Work out the finished part from the listing and answer in its coordinate system (mm). A direction names the side the tool comes from. Give positions to 0.01 mm unless a question says otherwise; leave off trailing zeros. Loops run counter-clockwise (first coordinate to the right, second up) from the corner with the lowest first, then second, coordinate; pieces in that order, holes last. Notation, with made-up numbers: M 63.5,-39 L 92.5,-39 A32 ccw 92.5,-4 Z; hole C 30,-4 d6. An arc over 180 degrees is marked long. Answer as a JSON object with one key per item and string values. Group by question number.
```python
from build123d import *

# Parameters (mm, degrees)
BOSS_EXTRUDE1_DEPTH     = 46.1
CUT_EXTRUDE1_START      = -8
CUT_EXTRUDE1_DEPTH      = 35.707069821
SKETCH3_R               = 5
CUT_EXTRUDE2_DEPTH      = 4.2
SKETCH4_R               = 3
CUT_EXTRUDE3_DEPTH      = 118.073974259
CUT_EXTRUDE4_START      = -33.042265264
CUT_EXTRUDE4_DEPTH      = 39.042265264
CUT_EXTRUDE4_START_2    = 14
CUT_EXTRUDE4_2_DEPTH    = 32.1
CUT_EXTRUDE4_START_3    = -47.726546034
CUT_EXTRUDE4_3_DEPTH    = 7.708156307
SKETCH8_W               = 31
SKETCH8_H               = 27.1
CUT_EXTRUDE5_DEPTH      = 119.273474775
SKETCH9_W               = 8
SKETCH9_H               = 25
BOSS_EXTRUDE2_DEPTH     = 19
SKETCH10_R              = 7.1
CUT_EXTRUDE6_DEPTH      = 119.273474775
SKETCH11_R              = 7.6
CUT_EXTRUDE7_DEPTH      = 1.2
CUT_EXTRUDE8_DEPTH      = 119.273474775
CUT_EXTRUDE8_DEPTH_BACK = 119.273474775
SKETCH12_R              = 2.1
CUT_EXTRUDE9_DEPTH      = 4.2
CUT_EXTRUDE9_DEPTH_BACK = 119.273474775
CUT_EXTRUDE9_START      = -8
SKETCH14_R              = 4
SKETCH14_R_2            = 2.1
CUT_EXTRUDE10_START     = -24
SKETCH14_3_R            = 4
CUT_EXTRUDE10_DEPTH     = 4.2
FILLET13_R              = 10
FILLET14_R              = 1


with BuildPart() as part:
    # Sketch1 → Boss-Extrude1 (new body)
    with BuildSketch(Plane(origin=(0, 0, 0), x_dir=(1, 0, 0), z_dir=(0, 1, 0))):
        with BuildLine():
            Line((0, 0), (8, 0))
            Line((8, 0), (8, -52.240297657))
            ThreePointArc((8, -52.240297657), (7.396926208, -55.660499091), (5.660444431, -58.668173754))
            Line((5.660444431, -58.668173754), (-19.707069821, -88.9))
            Line((-19.707069821, -88.9), (-19.707069821, -102.9))
            Line((-19.707069821, -102.9), (-27.707069821, -102.9))
            Line((-27.707069821, -102.9), (-27.707069821, -88.9))
            Line((-27.707069821, -88.9), (-2.339555569, -58.668173754))
            ThreePointArc((-2.339555569, -58.668173754), (-0.603073792, -55.660499091), (0, -52.240297657))
            Line((0, -52.240297657), (0, 0))
        make_face()
    extrude(amount=BOSS_EXTRUDE1_DEPTH)

    # Cut-Extrude1: read off the stored shape, not the designer's step
    # Cut-Extrude1 outline → Cut-Extrude1 (cut)
    with BuildSketch(Plane(origin=(-19.707069821, 0, 0), x_dir=(0, 0, -1), z_dir=(1, 0, 0)).offset(CUT_EXTRUDE1_START)):
        with BuildLine():
            ThreePointArc((-95.9, 0), (-100.849747468, 2.050252532), (-102.9, 7))
            Line((-102.9, 7), (-102.9, 0))
            Line((-102.9, 0), (-95.9, 0))
        make_face()
        with BuildLine():
            ThreePointArc((-102.9, 7), (-100.849747468, 11.949747468), (-95.9, 14))
            Line((-95.9, 14), (-88.9, 14))
            Line((-88.9, 14), (-88.852375001, 46.1))
            Line((-88.852375001, 46.1), (-102.9, 46.1))
            Line((-102.9, 46.1), (-102.9, 7))
        make_face()
    extrude(amount=CUT_EXTRUDE1_DEPTH, mode=Mode.SUBTRACT)

    # Sketch3 → Cut-Extrude2 (cut)
    with BuildSketch(Plane.ZY.offset(27.707069821)):
        with Locations((95.9, 7)):
            Circle(SKETCH3_R)
    extrude(amount=-CUT_EXTRUDE2_DEPTH, mode=Mode.SUBTRACT)

    # Sketch4 → Cut-Extrude3 (cut, through all)
    with BuildSketch(Plane.ZY.offset(23.507069821)):
        with Locations((95.9, 7)):
            Circle(SKETCH4_R)
    extrude(amount=-CUT_EXTRUDE3_DEPTH, mode=Mode.SUBTRACT)

    # Cut-Extrude4: read off the stored shape, not the designer's step
    # Cut-Extrude4 outline → Cut-Extrude4 (cut)
    with BuildSketch(Plane(origin=(-51.917191151, 0, 61.872499072), x_dir=(0.7660444431189772, 0, 0.6427876096865404), z_dir=(-0.6427876096865403, 0, 0.7660444431189771)).offset(CUT_EXTRUDE4_START)):
        Polygon((35.918971629, 46.1), (35.918971629, 14), (40.047327174, 46.1), align=None)
    extrude(amount=CUT_EXTRUDE4_DEPTH, mode=Mode.SUBTRACT)

    # Cut-Extrude4 2 outline → Cut-Extrude4 2 (cut)
    with BuildSketch(Plane(origin=(0, 0, 0), x_dir=(1, 0, 0), z_dir=(0, 1, 0)).offset(CUT_EXTRUDE4_START_2)):
        with BuildLine():
            Line((-3.162503825, -59.648925294), (0, -62.302581087))
            Line((0, -62.302581087), (0, -52.240297657))
            ThreePointArc((0, -52.240297657), (-0.603073792, -55.66049909), (-2.339555569, -58.668173754))
            Line((-2.339555569, -58.668173754), (-3.162503825, -59.648925294))
        make_face()
    extrude(amount=CUT_EXTRUDE4_2_DEPTH, mode=Mode.SUBTRACT)

    # Cut-Extrude4 3 outline → Cut-Extrude4 3 (add)
    with BuildSketch(Plane(origin=(0, 0, 0), x_dir=(0.7660444431189768, 0, 0.6427876096865408), z_dir=(0.6427876096865408, 0, -0.7660444431189768)).offset(CUT_EXTRUDE4_START_3)):
        Polygon((40.047327174, -46.1), (40.047327174, -14), (35.918971629, -14), align=None)
    extrude(amount=CUT_EXTRUDE4_3_DEPTH)

    # Sketch8 → Cut-Extrude5 (cut, through all)
    with BuildSketch(Plane(origin=(8, 0, 0), x_dir=(0, 0, -1), z_dir=(1, 0, 0))):
        with Locations((-15.5, 32.55)):
            Rectangle(SKETCH8_W, SKETCH8_H)
    extrude(amount=-CUT_EXTRUDE5_DEPTH, mode=Mode.SUBTRACT)

    # Sketch9 → Boss-Extrude2 (add)
    with BuildSketch(Plane(origin=(0, 0, 0), x_dir=(1, 0, 0), z_dir=(0, 1, 0))):
        with Locations((4, 12.5)):
            Rectangle(SKETCH9_W, SKETCH9_H)
    extrude(amount=BOSS_EXTRUDE2_DEPTH)

    # Sketch10 → Cut-Extrude6 (cut, through all)
    with BuildSketch(Plane(origin=(8, 0, 0), x_dir=(0, 0, -1), z_dir=(1, 0, 0))):
        with BuildLine():
            ThreePointArc((25, 3.947892292), (23.353975422, 1.740233099), (21.219790616, 0))
            Line((21.219790616, 0), (25, 0))
            Line((25, 0), (25, 3.947892292))
        make_face()
        with BuildLine():
            ThreePointArc((21.286823186, 18.957545444), (23.381362589, 17.231063475), (25, 15.052107708))
            Line((25, 15.052107708), (25, 19))
            Line((25, 19), (21.313922252, 19))
            Line((21.313922252, 19), (21.286823186, 18.957545444))
        make_face()
        with Locations((15.25, 9.5)):
            Circle(SKETCH10_R)
    extrude(amount=-CUT_EXTRUDE6_DEPTH, mode=Mode.SUBTRACT)

    # Sketch11 → Cut-Extrude7 (cut)
    with BuildSketch(Plane(origin=(8, 0, 0), x_dir=(0, 0, -1), z_dir=(1, 0, 0))):
        with Locations((15.25, 9.5)):
            Circle(SKETCH11_R)
    extrude(amount=-CUT_EXTRUDE7_DEPTH, mode=Mode.SUBTRACT)

    # Sketch12 → Cut-Extrude8 (cut, two sides: drawn at the far end of the back side and taken through both)
    with BuildSketch(Plane(origin=(8, 0, 0), x_dir=(0, 0, -1), z_dir=(1, 0, 0)).offset(-CUT_EXTRUDE8_DEPTH_BACK)):
        with Locations((-70.9, 5)):
            Circle(SKETCH12_R)
        with Locations((-10.9, 5)):
            Circle(SKETCH12_R)
    extrude(amount=CUT_EXTRUDE8_DEPTH + CUT_EXTRUDE8_DEPTH_BACK, mode=Mode.SUBTRACT)

    # Sketch14 → Cut-Extrude9 (cut, two sides: drawn at the far end of the back side and taken through both)
    with BuildSketch(Plane(origin=(8, 0, 0), x_dir=(0, 0, -1), z_dir=(1, 0, 0)).offset(CUT_EXTRUDE9_START - CUT_EXTRUDE9_DEPTH_BACK)):
        with Locations((-10.9, 5)):
            Circle(SKETCH14_R)
        with Locations((-10.9, 5)):
            Circle(SKETCH14_R_2, mode=Mode.SUBTRACT)
    extrude(amount=CUT_EXTRUDE9_DEPTH + CUT_EXTRUDE9_DEPTH_BACK, mode=Mode.SUBTRACT)

    # Sketch14<3> → Cut-Extrude10 (cut)
    with BuildSketch(Plane(origin=(8, 0, 0), x_dir=(0, 0, -1), z_dir=(1, 0, 0)).offset(CUT_EXTRUDE10_START)):
        with Locations((-70.9, 5)):
            Circle(SKETCH14_3_R)
    extrude(amount=CUT_EXTRUDE10_DEPTH, mode=Mode.SUBTRACT)

    # Fillet13
    # the kernel refuses this fillet: 10 mm, written as the material it adds along each edge
    with BuildSketch(Plane(origin=(-27.707069821, 14, 88.9), x_dir=(0, 0.9999988994008282, -0.0014836431957626689), z_dir=(1, 0, 0))) as fillet13_piece_1_section:
        with BuildLine():
            CenterArc((9.720956062, 10), FILLET13_R, 190.199837756, 79.800162244)
            Line((-0.121005032, 8.229180466), (-1.105201142, 8.052098513))
            ThreePointArc((-1.105201142, 8.052098513), (-1.010384402, 6.998508652), (-0.999998899, -0.001483643))
            Line((-0.999998899, -0.001483643), (0, -1))
            Line((0, -1), (9.720956062, -1))
            Line((9.720956062, -1), (9.720956062, 0))
        make_face()
    fillet13_piece_1 = extrude(amount=8, mode=Mode.PRIVATE)
    fillet13_piece_1 = split(fillet13_piece_1, bisect_by=Plane(origin=(-27.707069822, 14, 88.9), z_dir=(0.75978665319281, -0.12755860295201663, 0.6375367004675092)), keep=Keep.TOP, mode=Mode.PRIVATE)
    fillet13_piece_1 = split(fillet13_piece_1, bisect_by=Plane(origin=(-27.707069821, 14, 88.9), z_dir=(0.7660444431189771, 0, 0.6427876096865404)), keep=Keep.TOP, mode=Mode.PRIVATE)
    fillet13_piece_1 = split(fillet13_piece_1, bisect_by=Plane(origin=(-23.012477111, 14, 92.839231012), z_dir=(-0.7660444431189769, 0, -0.6427876096865407)), keep=Keep.TOP, mode=Mode.PRIVATE)
    add(fillet13_piece_1)
    with BuildSketch(Plane(origin=(-27.707069821, 14, 88.9), x_dir=(0, 0.9999988994008282, -0.0014836431957626689), z_dir=(1, 0, 0))) as fillet13_piece_2_section:
        with BuildLine():
            CenterArc((9.720956062, 10), FILLET13_R, 190.199837756, 79.800162244)
            Line((-0.121005032, 8.229180466), (-1.105201142, 8.052098513))
            ThreePointArc((-1.105201142, 8.052098513), (-1.010384402, 6.998508652), (-0.999998899, -0.001483643))
            Line((-0.999998899, -0.001483643), (0, -1))
            Line((0, -1), (9.720956062, -1))
            Line((9.720956062, -1), (9.720956062, 0))
        make_face()
    fillet13_piece_2 = extrude(amount=8, mode=Mode.PRIVATE)
    fillet13_piece_2 = split(fillet13_piece_2, bisect_by=Plane(origin=(-23.012477111, 14, 92.839231012), z_dir=(0.7660444431189769, 0, 0.6427876096865407)), keep=Keep.TOP, mode=Mode.PRIVATE)
    add(fillet13_piece_2)
    with BuildSketch(Plane(origin=(-27.707069821, 14, 88.9), x_dir=(0, 0.9999988994008282, -0.0014836431957626689), z_dir=(1, 0, 0))) as fillet13_piece_3_section:
        with BuildLine():
            CenterArc((9.720956062, 10), FILLET13_R, 190.199837756, 79.800162244)
            Line((-0.121005032, 8.229180466), (-1.105201142, 8.052098513))
            ThreePointArc((-1.105201142, 8.052098513), (-1.010384402, 6.998508652), (-0.999998899, -0.001483643))
            Line((-0.999998899, -0.001483643), (0, -1))
            Line((0, -1), (9.720956062, -1))
            Line((9.720956062, -1), (9.720956062, 0))
        make_face()
    fillet13_piece_3 = extrude(amount=32.302390155, mode=Mode.PRIVATE)
    fillet13_piece_3 = split(fillet13_piece_3, bisect_by=Plane(origin=(-19.707069821, 14, 88.9), z_dir=(1, 0, 0)), keep=Keep.TOP, mode=Mode.PRIVATE)
    fillet13_piece_3 = split(fillet13_piece_3, bisect_by=Plane(origin=(-23.012477111, 14, 92.839231012), z_dir=(-0.7660444431189769, 0, -0.6427876096865407)), keep=Keep.TOP, mode=Mode.PRIVATE)
    add(fillet13_piece_3)

    # Fillet14
    # the kernel refuses this fillet: 1 mm, written as the material it takes off along each edge
    with BuildSketch(Plane(origin=(6.8, 9.5, -15.25), x_dir=(0, 0, -1), z_dir=(0, -1, 0))) as fillet14_piece_1:
        with BuildLine():
            CenterArc((8.1, -0.866025404), FILLET14_R, 120, 60)
            Line((7.1, -0.866025404), (7.08, -0.866025404))
            Line((7.08, -0.866025404), (7.08, 0))
            Line((7.08, 0), (7.1, 0.02))
            ThreePointArc((7.1, 0.02), (7.35, 0.02), (7.59, 0.017320508))
            Line((7.59, 0.017320508), (7.6, 0))
        make_face()
    revolve(axis=Axis((6.8, 9.5, -15.25), (1, 0, 0)), mode=Mode.SUBTRACT)


solid = part.part
```
Item 1: A cutting plane is placed at A-A (z = 10.9). Determine the outline of the cut face in (x, y).
Item 2: For a pull along Z with two mould halves and no side action, classify faces 5 (the cylindrical face through (3.01, 2.57, -13.71)), 6 (the flat face through (2, 0, 37)), 7 (the cylindrical face through (7.414, 22.727, 55.615)) as pulls with the +Z half, pulls with the -Z half, needs draft (parallel to the pull), parting line crosses it, or undercut.
Item 3: A cutting plane is placed at D-D (x = -17.5). Determine the outline of the cut face in (y, z).
Item 4: Find the intervals of material crossed by probe 1 along Y at (x, z) = (1.5, -15.25); probe 2 along Z at (x, y) = (6.05, 5); probe 3 along Z at (x, y) = (1.45, 5), in increasing order. Write a range as [from, to].
Item 5: A tool of negligible diameter and unlimited length cuts with its end or side. For faces 1 (the flat face through (-0.4, 14, 55.7)), 2 (the flat face through (4, 32, 31)), 3 (the flat face through (-19.707, 9, 93)), 4 (the cylindrical face through (2.071, 1.095, 11.767)), from which of +Z, -Z, +X, -X, +Y, -Y can it reach the whole face along a straight path? Write none if from no direction.
Item 6: A cutting plane is placed at C-C (z = -15.25). Determine the outline of the cut face in (x, y).
Item 7: Given pin 1 Ø3 at (x, y) = (1.5, 23) entering from +Z; pin 2 Ø9 at (y, z) = (7, 95.9) entering from -X; pin 3 Ø2.5 at (y, z) = (6, 10) entering from -X, each flat-ended and moving along its own axis, determine where each tip first touches the part or whether it passes through.
Item 8: A cutting plane is placed at B-B (y = 31). Determine the outline of the cut face in (x, z).
The answers:
{
 "1": {"outline": "M 0,0 L 8,0 L 8,2.9 L 4.2,2.9 L 4.2,1 L 0,1 Z; M 0,9 L 4.2,9 L 4.2,7.1 L 8,7.1 L 8,19 L 0,19 Z"},
 "2": {"face 5": "undercut", "face 6": "needs draft", "face 7": "pulls with the +Z half"},
 "3": {"outline": "M 0,76.74 L 14,76.74 L 46.1,83.16 L 46.1,86.27 L 0,86.27 Z"},
 "4": {"probe 1": "y = [0, 2.4], [16.6, 19]", "probe 2": "z = [-25, -20.75], [-9.75, 8.8], [13, 58.17]", "probe 3": "z = [-25, -20.74], [-9.76, 6.9], [14.9, 63.69]"},
 "5": {"face 1": "-Z, -X, +Y", "face 2": "-Z, +X, -X, +Y", "face 3": "+Z, +X, +Y, -Y", "face 4": "-X"},
 "6": {"outline": "M 0,0 L 8,0 L 8,1.9 L 6.8,1.9 A1 ccw 5.93,2.4 L 0,2.4 Z; M 0,16.6 L 5.93,16.6 A1 ccw 6.8,17.1 L 8,17.1 L 8,19 L 0,19 Z"},
 "7": {"pin 1": "stops at z = 65.41", "pin 2": "stops at x = -23.51", "pin 3": "stops at x = 4.2"},
 "8": {"outline": "M -24.83,88.87 L 0,59.28 L 0,31 L 8,31 L 8,52.24 A10 ccw 5.66,58.67 L -19.69,88.87 Z"}
}
